Input: part model. Units: mm. Frame: model coordinates. Face numbers are marked on the shaded views. A direction names the side the tool comes from. Coordinates: 2 decimals unless noted, no trailing zeros. Loops run counter-clockwise (first coordinate to the right, second up) from the corner with the lowest first, then second, coordinate; pieces in that order, holes last. Notation, with made-up numbers: M -33.75,20.25 L -9.75,20.25 A18 cw -9.75,39.25 Z; hole C 60.5,29.5 d1. An arc over 180 degrees is marked long. Use a Markdown table: item, result. Add a question column.
1. Line query: L1, parallel to Z at x = 1, y = 47.5; L2, parallel to X at y = 67, z = 0; L3, parallel to Y at x = -23.5, z = -9. Output: solid intervals per line, ascending. Write a range as [from, to].
2. Pin query (flat end, axial travel): pin 1 (10 mm diameter, centred on x = -14.5, z = -8, fed in from +Y); pin 2 (15.5 mm diameter, centred on x = 20, z = -34.64, fed in from -Y); pin 3 (3 mm diameter, centred on x = 27.5, y = 30.5, fed in from +Z); pin 4 (6 mm diameter, centred on x = 15.5, y = 18.5, fed in from +Z). Return the tip coordinate at first contact, or that it passes through.
3. Section B-B on z = 0. Output: boundary loops of the cut face in (x, y), then the cut area to 3 significant figures.
4. Section C-C on z = -35. Output: boundary loops of the cut face in (x, y), then the cut area to 3 significant figures.
5. Section D-D on x = -40. Output: boundary loops of the cut face in (y, z).
6. Set-up query: the marked faces 1 and 2. Return all of +Z, -Z, +X, -X, +Y, -Y with unobstructed straight access to the full face (end or side cutting, diameter ignored); none if empty.
7. Section A-A on x = 0. Output: boundary loops of the cut face in (y, z), then the cut area to 3 significant figures.
8. Draft query along Y for the marked faces 3, 4 and 5. Return one class per face: +Y half, -Y half, draft (parallel to the pull), parting line (faces both ways), or undercut.
```python
from build123d import *

# Parameters (mm, degrees)
SKETCH2_R           = 30
BOSS_EXTRUDE1_DEPTH = 35
SKETCH3_R           = 25
BOSS_EXTRUDE2_DEPTH = 45
SKETCH4_R           = 50
BOSS_EXTRUDE3_DEPTH = 8
SKETCH5_R           = 25
CUT_EXTRUDE1_DEPTH  = 25
CUT_EXTRUDE2_REACH  = 90
SKETCH6_R           = 20
SKETCH7_R           = 5.9
CUT_EXTRUDE3_DEPTH  = 40
CIRPATTERN1_COUNT   = 6


with BuildPart() as part:
    # Sketch2 → Boss-Extrude1 (new body)
    with BuildSketch(Plane(origin=(0, 0, 0), x_dir=(1, 0, 0), z_dir=(0, 1, 0))):
        Circle(SKETCH2_R)
    extrude(amount=BOSS_EXTRUDE1_DEPTH)

    # Sketch3 → Boss-Extrude2 (add)
    with BuildSketch(Plane(origin=(0, 35, 0), x_dir=(1, 0, 0), z_dir=(0, 1, 0))):
        Circle(SKETCH3_R)
    extrude(amount=BOSS_EXTRUDE2_DEPTH)

    # Sketch4 → Boss-Extrude3 (add)
    with BuildSketch(Plane(origin=(0, 80, 0), x_dir=(1, 0, 0), z_dir=(0, 1, 0))):
        Circle(SKETCH4_R)
    extrude(amount=BOSS_EXTRUDE3_DEPTH)

    # Sketch5 → Cut-Extrude1 (cut)
    with BuildSketch(Plane.XZ):
        Circle(SKETCH5_R)
    extrude(amount=-CUT_EXTRUDE1_DEPTH, mode=Mode.SUBTRACT)

    # Sketch6 → Cut-Extrude2 (cut, up to next)
    with BuildSketch(Plane(origin=(0, 88, 0), x_dir=(1, 0, 0), z_dir=(0, 1, 0)), mode=Mode.PRIVATE) as cut_extrude2_sk1:
        Circle(SKETCH6_R)
    cut_extrude2_tool1 = extrude(cut_extrude2_sk1.sketch, amount=-CUT_EXTRUDE2_REACH, mode=Mode.PRIVATE) & part.part
    add(cut_extrude2_tool1.solids().sort_by_distance((0, 88, 0))[0], mode=Mode.SUBTRACT)

    # Sketch7 → Cut-Extrude3 (cut)
    with BuildSketch(Plane(origin=(0, 88, 0), x_dir=(1, 0, 0), z_dir=(0, 1, 0))):
        with Locations((40, 0)):
            Circle(SKETCH7_R)
    cut_extrude3 = extrude(amount=-CUT_EXTRUDE3_DEPTH, mode=Mode.SUBTRACT)

    # CirPattern1: Cut-Extrude3 ×6 about axis
    cirpattern1_axis = Axis((0, 0, 0), (0, 1, 0))
    for i in range(1, CIRPATTERN1_COUNT):
        add(cut_extrude3.rotate(cirpattern1_axis, i * 360 / CIRPATTERN1_COUNT), mode=Mode.SUBTRACT)


solid = part.part
```
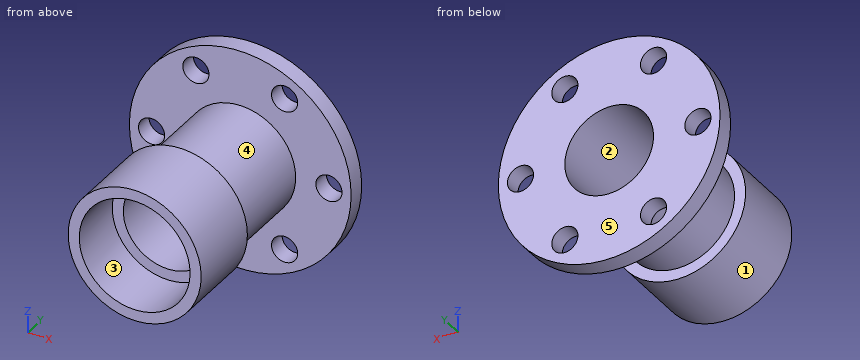
Answers below:
| question | item | result |
|---|---|---|
| 1 | L1 | z = [-24.98, -19.97], [19.97, 24.98] |
| 1 | L2 | x = [-25, -20], [20, 25] |
| 1 | L3 | y = [0, 35], [80, 88] |
| 2 | pin 1 | stops at y = 88 |
| 2 | pin 2 | stops at y = 80 |
| 2 | pin 3 | stops at z = 14.97 |
| 2 | pin 4 | stops at z = 27.27 |
| 3 | outline | M -50,80 L -45.9,80 L -45.9,88 L -50,88 Z; M -34.1,80 L -25,80 L -25,35 L -30,35 L -30,0 L -25,0 L -25,25 L -20,25 L -20,88 L -34.1,88 Z; M 20,25 L 25,25 L 25,0 L 30,0 L 30,35 L 25,35 L 25,80 L 34.1,80 L 34.1,88 L 20,88 Z; M 45.9,80 L 50,80 L 50,88 L 45.9,88 Z |
| 3 | area | 1,190 mm² |
| 4 | outline | M -35.71,80 L -25.89,80 L -25.89,88 L -35.71,88 Z; M -14.11,80 L 14.11,80 L 14.11,88 L -14.11,88 Z; M 25.89,80 L 35.71,80 L 35.71,88 L 25.89,88 Z |
| 4 | area | 383 mm² |
| 5 | outline | M 80,-30 L 88,-30 L 88,-5.9 L 80,-5.9 Z; M 80,5.9 L 88,5.9 L 88,30 L 80,30 Z |
| 6 | face 1 | -Y |
| 6 | face 2 | +Y, -Y |
| 7 | outline | M 0,-30 L 35,-30 L 35,-25 L 80,-25 L 80,-50 L 88,-50 L 88,-20 L 25,-20 L 25,-25 L 0,-25 Z; M 0,25 L 25,25 L 25,20 L 88,20 L 88,50 L 80,50 L 80,25 L 35,25 L 35,30 L 0,30 Z |
| 7 | area | 1,380 mm² |
| 8 | face 3 | draft |
| 8 | face 4 | undercut |
| 8 | face 5 | +Y half |
